Geometry check sheet. Reference: the model listing, model coordinates, mm. Face numbers are marked on the shaded views. A direction names the side the tool comes from. Give positions to 0.01 mm unless a question says otherwise; leave off trailing zeros. Order: outer loops, then holes, each group sorted by start corner. A loop starts at its lowest first (then second) coordinate and runs counter-clockwise, first axis right, second up.
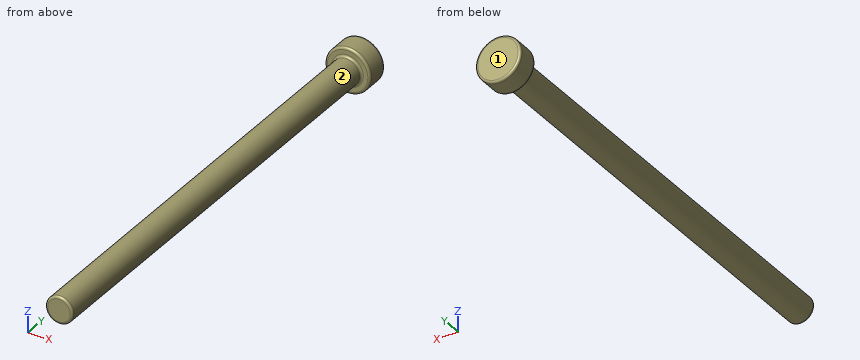
from build123d import *

# Parameters (mm, degrees)
SKETCH_1_R      = 5
EXTRUDE_1_DEPTH = 5
SKETCH_2_R      = 3
EXTRUDE_2_DEPTH = 100
FILLET_1_R      = 0.5


with BuildPart() as part:
    # 草圖1 → 伸長1 (new body)
    with BuildSketch(Plane(origin=(0, 0, 0), x_dir=(1, 0, 0), z_dir=(0, 1, 0))):
        with Locations(Location((0, 0, 0), (0, 0, 270))):
            Circle(SKETCH_1_R)
    extrude(amount=EXTRUDE_1_DEPTH)

    # 草圖2 → 伸長2 (add)
    with BuildSketch(Plane.XZ):
        with Locations(Location((0, 0, 0), (0, 0, 90))):
            Circle(SKETCH_2_R)
    extrude(amount=EXTRUDE_2_DEPTH)

    # 圓角1
    fillet_1_edges = [part.edges().sort_by_distance(p)[0] for p in [
        (0, 0, -5),
        (0, 5, -5),
        (0, 0, -3),
        (0, -100, -3),
    ]]
    fillet(fillet_1_edges, radius=FILLET_1_R)


solid = part.part
Item 1: Scan lines: L1, parallel to Y at x = 3.75, z = -2; L2, parallel to Z at x = -0.25, y = -40.5. Record each from-to range of solid material in increasing order.
Reported:
L1: y = 0 to 5
L2: z = -2.99 to 2.99
Item 2: Set-up check for the marked faces 1 and 2: record each of +Z, -Z, +X, -X, +Y, -Y from which the full face is reachable in a straight line by a thin tool's end or side.
Reported:
face 1: +Z, -Z, +X, -X, +Y
face 2: -Y
Item 3: Gauge pin test, flat ends, axial feed: pin 1 (4 mm diameter, centred on y = -47.5, z = 0, fed in from -X); pin 2 (2 mm diameter, centred on x = 1, y = -56.5, fed in from +Z); pin 3 (5 mm diameter, centred on y = -21, z = -2, fed in from +X). Record the tip position at first contact, or that the pin passes through.
Reported:
pin 1: stops at x = -3
pin 2: stops at z = 3
pin 3: stops at x = 3
Item 4: Sectioned sample at A-A (x = 0). Enter the section's corners in (y, z).
Reported:
outline: (-100, -2.5) arc R0.5 ccw to (-99.5, -3) - (-0.5, -3) arc R0.5 cw to (0, -3.5) - (0, -4.5) arc R0.5 ccw to (0.5, -5) - (4.5, -5) arc R0.5 ccw to (5, -4.5) - (5, 4.5) arc R0.5 ccw to (4.5, 5) - (0.5, 5) arc R0.5 ccw to (0, 4.5) - (0, 3.5) arc R0.5 cw to (-0.5, 3) - (-99.5, 3) arc R0.5 ccw to (-100, 2.5) - close
Item 5: Sectioned sample at C-C (y = -33.5). Enter the section's corners in (x, z), and give its area (3 significant figures).
Reported:
outline: circle Ø6 at (0, 0)
area: 28.3 mm2
Item 6: Sectioned sample at B-B (z = 0). Enter the section's corners in (x, y), and give its area (3 significant figures).
Reported:
outline: (-5, 0.5) arc R0.5 ccw to (-4.5, 0) - (-3.5, 0) arc R0.5 cw to (-3, -0.5) - (-3, -99.5) arc R0.5 ccw to (-2.5, -100) - (2.5, -100) arc R0.5 ccw to (3, -99.5) - (3, -0.5) arc R0.5 cw to (3.5, 0) - (4.5, 0) arc R0.5 ccw to (5, 0.5) - (5, 4.5) arc R0.5 ccw to (4.5, 5) - (-4.5, 5) arc R0.5 ccw to (-5, 4.5) - close
area: 650 mm2
